Autodesk Inventor part; units mm, degrees
ref_plane "YZ Plane" through (0, 0, 0) normal (1, 0, 0) x (0, 1, 0)
ref_plane "XZ Plane" through (0, 0, 0) normal (0, 1, 0) x (-1, 0, 0)
ref_plane "XY Plane" through (0, 0, 0) normal (0, 0, 1) x (1, 0, 0)
sketch "Sketch1" plane through (0, 0, 0) normal (0, 1, 0) x (-1, 0, 0)
  line L0 (0, 0) -> (59.4, 0)
  line L1 (59.4, 0) -> (59.4, -59.4)
  line L2 (59.4, -59.4) -> (0, -59.4)
  line L3 (0, -59.4) -> (0, 0)
  dimension "d0" = 59.4
  dimension "d1" = 59.4
extrude "Extrusion1" add sketch "Sketch1" along normal blind 18.1
sketch "Sketch2" plane through (0, 18.1, 0) normal (0, 1, 0) x (1, 0, 0)
  line L0 (-59.4, 59.4) -> (-59.4, 0)
  line L1 (-59.4, 29.7) -> (0, 29.7)
  line L2 (-29.7, 29.7) -> (-29.7, 59.4)
  line L3 (-29.7, 29.7) -> (-29.7, 17)
  circle A0 centre (-29.7, 17) radius 5.08
  line L4 (-29.7, 17) -> (-42.4, 17)
  line L5 (-29.7, 17) -> (-17, 17)
  circle A1 centre (-42.4, 17) radius 5.08
  circle A2 centre (-17, 17) radius 5.08
  line L6 (-29.7, 29.7) -> (-29.7, 42.4)
  circle A3 centre (-29.7, 42.4) radius 5.08
  line L7 (-29.7, 42.4) -> (-42.4, 42.4)
  line L8 (-29.7, 42.4) -> (-17, 42.4)
  circle A4 centre (-42.4, 42.4) radius 5.08
  circle A5 centre (-17, 42.4) radius 5.08
  circle A6 centre (-29.7, 17) radius 3.175
  circle A7 centre (-42.4, 17) radius 3.175
  circle A8 centre (-17, 17) radius 3.175
  circle A9 centre (-29.7, 42.4) radius 3.175
  circle A10 centre (-42.4, 42.4) radius 3.175
  circle A11 centre (-17, 42.4) radius 3.175
  circle A12 centre (-29.7, 29.7) radius 3.175
  line L9 (-29.7, 29.7) -> (-29.7, 34.704)
  line L10 (-29.7, 29.7) -> (-29.7, 24.696)
  circle A13 centre (-29.7, 24.696) radius 1.0125
  circle A14 centre (-29.7, 34.704) radius 1.0125
  point P0 (0, 0)
  dimension "d4" = 12.7
  dimension "d5" = 10.16
  dimension "d6" = 12.7
  dimension "d7" = 12.7
  dimension "d8" = 10.16
  dimension "d9" = 10.16
  dimension "d10" = 12.7
  dimension "d11" = 10.16
  dimension "d12" = 12.7
  dimension "d13" = 12.7
  dimension "d14" = 10.16
  dimension "d15" = 10.16
  dimension "d16" = 6.35
  dimension "d17" = 6.35
  dimension "d18" = 6.35
  dimension "d19" = 6.35
  dimension "d20" = 6.35
  dimension "d21" = 6.35
  dimension "d22" = 6.35
  dimension "d23" = 5.004
  dimension "d24" = 5.004
  dimension "d25" = 2.025
  dimension "d26" = 2.025
extrude "Extrusion2" cut sketch "Sketch2" against normal blind 38.1 contours L2 A12 L1 | L3 A12 L1 | L1 A12 L2 | L1 A12 L3 | A8 | A7 | A10 | A11 | A9 L7 L2 | L2 L8 A9 | A6 L5 L3 | L3 L4 A6 | L7 A9 L2 | L2 A9 L8 | L5 A6 L4
extrude "Extrusion3" cut sketch "Sketch2" against normal blind 7.62 contours A8 | A2 | A7 | A1 | A0 L5 A6 L3 | L3 A6 L4 A0 | A4 | A11 | A5 | A3 L7 A9 L2 | L2 A9 L8 A3 | A9 L7 L2 | L2 L8 A9 | A3 L2 A9 L7 | L8 A9 L2 A3 | A6 L5 L3 | L3 L4 A6 | A0 L4 A6 L5 | L7 A9 L2 | L2 A9 L8 | L5 A6 L4
extrude "Extrusion4" cut sketch "Sketch2" against normal blind 4.445 contours A13 L3 | L3 A13 | A14 L2 | L2 A14
sketch "Sketch3" plane through (0, 0, 0) normal (0, -1, 0) x (1, 0, 0)
  circle A0 centre (-29.7, -29.7) radius 3.175
  line L0 (-29.7, -29.7) -> (-29.7, -51.7)
  line L1 (-29.7, -29.7) -> (-29.7, -7.7)
  circle A1 centre (-29.7, -7.7) radius 1.5125
  circle A2 centre (-29.7, -51.7) radius 1.5125
  circle A3 centre (-29.7, -29.7) radius 5.08
  point P0 (0, 0)
  dimension "d33" = 22
  dimension "d34" = 22
  dimension "d35" = 3.025
  dimension "d36" = 3.025
  dimension "d37" = 10.16
extrude "Extrusion5" cut sketch "Sketch3" against normal blind 4.445 contours A1 | A2
extrude "Extrusion6" cut sketch "Sketch3" against normal blind 7.62 contours A0 L0 L1 | A0 L1 A3 L0 | L1 L0 A0 | A0 L0 A3 L1
fillet "Fillet1" radius 3.175 4 edges at (0, 9.05, -59.4) (0, 9.05, 0) (-59.4, 9.05, 0) (-59.4, 9.05, -59.4)
properties part number "LNR25MtoPolarisAdapter"
Part model, mm, in its own coordinate system. A direction names the side the tool comes from. Round coordinates to 2 decimals unless told otherwise and drop trailing zeros. Order: outer loops, then holes, each group sorted by start corner. A loop starts at its lowest first (then second) coordinate and runs counter-clockwise, first axis right, second up. Notation, with made-up numbers: M 73,66.25 L 118,66.25 A23 cw 118,79.25 Z; hole C 78.5,-17.75 d6. An arc over 180 degrees is marked long. Answer in a Markdown table with one row per item. Add a question column.
Q1. Cut at A-A on x = -17. Give the cut face in (y, z) (3 decimals), and give its area (3 significant figures).
Q2. Mould opens along Z. For faces 4 (the face through (-0.95, 9.18, -0.91)), 5 (the face through (-29, 18.1, -23)), 6 (the face through (-15.293, 5.313, -45.077)) say: +Z half, -Z half, draft (parallel to the pull), parting line (faces both ways), or undercut.
Q3. Cut at B-B on z = -42.4. Give the cut face in (x, y) (3 decimals), and give its area (3 significant figures).
Q4. Pin check, flat tips, straight feed: pin 1 (9 mm diameter, centred on x = -42.4, z = -17, fed in from +Y); pin 2 (2.5 mm diameter, centred on x = -29.7, z = -7.7, fed in from -Y) (3 decimals). Stop position of each tip, or through.
Q5. Wall check: L1, parallel to Z at x = -29.7, y = 2.95 (1 decimal); L2, parallel to Z at x = -29.7, y = 14 (1 decimal); L3, parallel to X at y = 13.5, z = -42.4. Give the ranges that are in metal, low to high. Write a range as from..to.
Q6. Cut at D-D on x = -27.5. Give the cut face in (y, z), and give its area (3 significant figures).
Q7. Cut at C-C on y = 9. Give the cut face in (x, z) (3 decimals), and give its area (3 significant figures).
Q8. 3-axis set-ups, long thin cutter, end or side, ignore diameter. For faces 1 (the face through (-30, 4.445, -8)), 2 (the face through (-30.11, 5.31, -20.15)), 3 (the face through (-17, 10.48, -39)): which of +Z, -Z, +X, -X, +Y, -Y reach the whole face in a straight line?
Established:
| question | item | result |
|---|---|---|
| 1 | outline | M 0,-59.4 L 18.1,-59.4 L 18.1,-47.48 L 10.48,-47.48 L 10.48,-45.575 L 0,-45.575 Z; M 0,-39.225 L 10.48,-39.225 L 10.48,-37.32 L 18.1,-37.32 L 18.1,-22.08 L 10.48,-22.08 L 10.48,-20.175 L 0,-20.175 Z; M 0,-13.825 L 10.48,-13.825 L 10.48,-11.92 L 18.1,-11.92 L 18.1,0 L 0,0 Z |
| 1 | area | 787 mm2 |
| 2 | face 4 | +Z half |
| 2 | face 5 | draft |
| 2 | face 6 | undercut |
| 3 | outline | M -59.4,0 L -45.575,0 L -45.575,10.48 L -47.48,10.48 L -47.48,18.1 L -59.4,18.1 Z; M -39.225,0 L -32.875,0 L -32.875,10.48 L -34.78,10.48 L -34.78,18.1 L -37.32,18.1 L -37.32,10.48 L -39.225,10.48 Z; M -26.525,0 L -20.175,0 L -20.175,10.48 L -22.08,10.48 L -22.08,18.1 L -24.62,18.1 L -24.62,10.48 L -26.525,10.48 Z; M -13.825,0 L 0,0 L 0,18.1 L -11.92,18.1 L -11.92,10.48 L -13.825,10.48 Z |
| 3 | area | 643 mm2 |
| 4 | pin 1 | stops at y = 10.48 |
| 4 | pin 2 | stops at y = 4.445 |
| 5 | L1 | z = -59.4..-53.2, -50.2..-45.6, -39.2..-34.8, -24.6..-20.2, -13.8..-9.2, -6.2..0 |
| 5 | L2 | z = -59.4..-47.5, -37.3..-35.7, -33.7..-32.9, -26.5..-25.7, -23.7..-22.1, -11.9..0 |
| 5 | L3 | x = -59.4..-47.48, -37.32..-34.78, -24.62..-22.08, -11.92..0 |
| 6 | outline | M 0,-59.4 L 18.1,-59.4 L 18.1,-46.98 L 10.48,-46.98 L 10.48,-44.69 L 0,-44.69 Z; M 0,-40.11 L 10.48,-40.11 L 10.48,-37.82 L 18.1,-37.82 L 18.1,-31.99 L 7.62,-31.99 L 7.62,-34.28 L 0,-34.28 Z; M 0,-25.12 L 7.62,-25.12 L 7.62,-27.41 L 18.1,-27.41 L 18.1,-21.58 L 10.48,-21.58 L 10.48,-19.29 L 0,-19.29 Z; M 0,-14.71 L 10.48,-14.71 L 10.48,-12.42 L 18.1,-12.42 L 18.1,0 L 0,0 Z |
| 6 | area | 722 mm2 |
| 7 | outline | M -59.4,-56.225 A3.175 ccw -56.225,-59.4 L -3.175,-59.4 A3.175 ccw 0,-56.225 L 0,-3.175 A3.175 ccw -3.175,0 L -56.225,0 A3.175 ccw -59.4,-3.175 Z; hole C -42.4,-42.4 d6.35; hole C -42.4,-17 d6.35; hole C -29.7,-42.4 d6.35; hole C -29.7,-29.7 d6.35; hole C -29.7,-17 d6.35; hole C -17,-42.4 d6.35; hole C -17,-17 d6.35 |
| 7 | area | 3,300 mm2 |
| 8 | face 1 | -Y |
| 8 | face 2 | +Y, -Y |
| 8 | face 3 | +Y |
